from build123d import *

# Parameters (mm, degrees)
SKETCH_1_W          = 56
SKETCH_1_H          = 25
EXTRUDE_1_DEPTH     = 44.5
CUT_EXTRUDE_1_DEPTH = 59.21726548
CUT_EXTRUDE_2_DEPTH = 73.611982482
SKETCH_4_R          = 4
SKETCH_4_R_2        = 1.5
CUT_EXTRUDE_3_DEPTH = 53.407060593
SKETCH_5_R          = 4
SKETCH_5_R_2        = 1.5
CUT_EXTRUDE_4_DEPTH = 73.611982482
FILLET_1_R          = 1


with BuildPart() as part:
    # 草图1 → 凸台-拉伸1 (new body)
    with BuildSketch(Plane.XY):
        Rectangle(SKETCH_1_W, SKETCH_1_H)
    extrude(amount=EXTRUDE_1_DEPTH)

    # 草图2 → 切除-拉伸1 (cut, through all)
    with BuildSketch(Plane.XZ.offset(12.5)):
        Polygon((0, 44.5), (26, 44.5), (26, 2), (-26, 2), (-26, 44.5), align=None)
    extrude(amount=-CUT_EXTRUDE_1_DEPTH, mode=Mode.SUBTRACT)

    # 草图3 → 切除-拉伸2 (cut, through all)
    with BuildSketch(Plane(origin=(28, 0, 0), x_dir=(0, 0, -1), z_dir=(1, 0, 0))):
        with BuildLine():
            ThreePointArc((-44.5, 0), (-40.838834765, 8.838834765), (-32, 12.5))
            Line((-32, 12.5), (-44.5, 12.5))
            Line((-44.5, 12.5), (-44.5, 0))
        make_face()
        with BuildLine():
            ThreePointArc((-32, -12.5), (-40.838834765, -8.838834765), (-44.5, 0))
            Line((-44.5, 0), (-44.5, -12.5))
            Line((-44.5, -12.5), (-32, -12.5))
        make_face()
    extrude(amount=-CUT_EXTRUDE_2_DEPTH, mode=Mode.SUBTRACT)

    # 草图4 → 切除-拉伸3 (cut, through all)
    with BuildSketch(Plane.XY.offset(2)):
        Circle(SKETCH_4_R)
        with Locations((0, 7)):
            Circle(SKETCH_4_R_2)
        with Locations((0, -7)):
            Circle(SKETCH_4_R_2)
        with Locations((-7, 0)):
            Circle(SKETCH_4_R_2)
        with Locations((7, 0)):
            Circle(SKETCH_4_R_2)
        with Locations((18.6, 0)):
            Circle(SKETCH_4_R_2)
        with Locations(Location((-18.6, 0, 0), (0, 0, 180))):
            Circle(SKETCH_4_R_2)
    extrude(amount=-CUT_EXTRUDE_3_DEPTH, mode=Mode.SUBTRACT)

    # 草图5 → 切除-拉伸4 (cut, through all)
    with BuildSketch(Plane(origin=(28, 0, 0), x_dir=(0, 0, -1), z_dir=(1, 0, 0))):
        with Locations((-32, 0.108344676)):
            Circle(SKETCH_5_R)
        with Locations((-32, 7.108344676)):
            Circle(SKETCH_5_R_2)
        with Locations((-39, 0.108344676)):
            Circle(SKETCH_5_R_2)
        with Locations((-32, -6.891655324)):
            Circle(SKETCH_5_R_2)
        with Locations((-25, 0.108344676)):
            Circle(SKETCH_5_R_2)
        with Locations((-13.4, 0.108344676)):
            Circle(SKETCH_5_R_2)
    extrude(amount=-CUT_EXTRUDE_4_DEPTH, mode=Mode.SUBTRACT)

    # 圆角1
    fillet_1_edges = [part.edges().sort_by_distance(p)[0] for p in [
        (26, 0, 2),
        (-26, 0, 2),
        (-28, 0, 0),
        (28, 0, 0),
    ]]
    fillet(fillet_1_edges, radius=FILLET_1_R)


solid = part.part
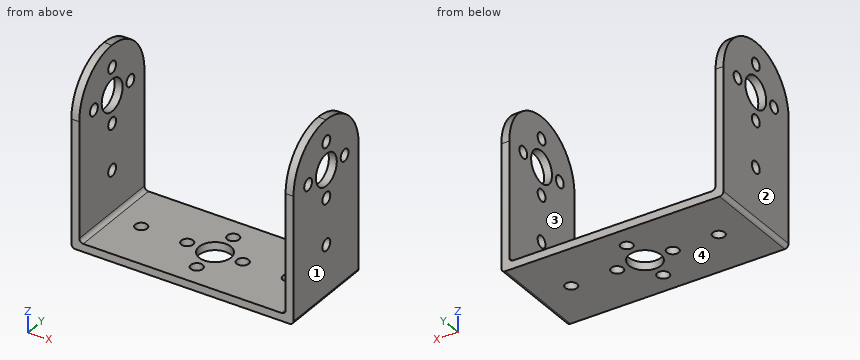
Here's how the part is built. I have some questions about the finished solid (model axes, mm). Face numbers are marked on the shaded views. Round coordinates to 2 decimals unless told otherwise and drop trailing zeros. Order: outer loops, then holes, each group sorted by start corner. A loop starts at its lowest first (then second) coordinate and runs counter-clockwise, first axis right, second up. Notation, with made-up numbers: (42, 7.25) -> (88, 7.25) arc R27 ccw to (88, 43.25) -> close; hole circle Ø11 at (15.25, -38). An arc over 180 degrees is marked (long way). Use CSV: the item, a comma, the result in double quotes.
1. I'm going to push flat-ended pins straight in: P1, Ø5, axis at y = 0.11, z = 32, coming from the -X side (3 decimals); P2, Ø3, axis at x = 2, y = -6, coming from the +Z side. Where does each tip first touch, or does it pass through?
Recorded:
P1,"passes through"
P2,"stops at z = 2"
2. I need wall thicknesses on line 1 along Y through (x, z) = (0, 1.55); line 2 along X through (y, z) = (-4.5, 15); line 3 along Y through (x, z) = (-18.6, 1.15). Which ranges of each line are inside material? Lowest first, please.
Recorded:
line 1,"y = -12.5 to -8.5, -5.5 to -4, 4 to 5.5, 8.5 to 12.5"
line 2,"x = -28 to -26, 26 to 28"
line 3,"y = -12.5 to -1.5, 1.5 to 12.5"
3. I want a section at D-D on y = -6.25. List the corners of the cut face in (x, z) for me.
Recorded:
outline,"(-28, 1) arc R1 ccw to (-27, 0) -> (-1.3, 0) -> (-1.3, 2) -> (-25, 2) arc R1 cw to (-26, 3) -> (-26, 30.64) -> (-28, 30.64) -> close; (-28, 33.36) -> (-26, 33.36) -> (-26, 42.83) -> (-28, 42.83) -> close; (1.3, 0) -> (27, 0) arc R1 ccw to (28, 1) -> (28, 30.64) -> (26, 30.64) -> (26, 3) arc R1 cw to (25, 2) -> (1.3, 2) -> close; (26, 33.36) -> (28, 33.36) -> (28, 42.83) -> (26, 42.83) -> close"
4. I want a section at A-A on x = 18.6. List the corners of the cut face in (y, z) for me, and give its area (3 significant figures).
Recorded:
outline,"(-12.5, 0) -> (-1.5, 0) -> (-1.5, 2) -> (-12.5, 2) -> close; (1.5, 0) -> (12.5, 0) -> (12.5, 2) -> (1.5, 2) -> close"
area,"44.0 mm2"
5. I want a section at B-B on z = 19.5. List the corners of the cut face in (x, y) for me, and give its area (3 significant figures).
Recorded:
outline,"(-28, -12.5) -> (-26, -12.5) -> (-26, 12.5) -> (-28, 12.5) -> close; (26, -12.5) -> (28, -12.5) -> (28, 12.5) -> (26, 12.5) -> close"
area,"100 mm2"
6. Thinking about a two-plate mould opening in X: for the marked faces 1, 2, 3 and 4, which applies, pulls with the +X half, pulls with the -X half, needs draft (parallel to the pull), parting line crosses it, or undercut?
Recorded:
face 1,"pulls with the +X half"
face 2,"pulls with the -X half"
face 3,"undercut"
face 4,"needs draft"
7. I want a section at C-C on z = 25. List the corners of the cut face in (x, y) for me, and give its area (3 significant figures).
Recorded:
outline,"(-28, -12.5) -> (-26, -12.5) -> (-26, -1.39) -> (-28, -1.39) -> close; (-28, 1.61) -> (-26, 1.61) -> (-26, 12.5) -> (-28, 12.5) -> close; (26, -12.5) -> (28, -12.5) -> (28, -1.39) -> (26, -1.39) -> close; (26, 1.61) -> (28, 1.61) -> (28, 12.5) -> (26, 12.5) -> close"
area,"88.0 mm2"
